Read the model definition and answer for the solid it produces. Units are mm, in the model's axes. Face numbers are marked on the shaded views. A direction names the side the tool comes from. Give positions to 0.01 mm unless a question says otherwise; leave off trailing zeros. Write each loop counter-clockwise with the first axis right and the second up, starting at its lowest first coordinate (ties: lowest second). Pieces come first, ordered by that corner, then holes. Notation, with made-up numbers: (45.5, 50.5) -> (101.5, 50.5) arc R26 cw to (101.5, 81.5) -> close; hole circle Ø6 at (-8, 85). An arc over 180 degrees is marked (long way). Answer as CSV lines item,"result". Start each with the question number.
1. For a pull along Y with two mould halves and no side action, classify the marked faces 3, 4 and 5 as pulls with the +Y half, pulls with the -Y half, needs draft (parallel to the pull), parting line crosses it, or undercut.
2. The part is cut by section A-A, the plane x = 0. Determine the outline of the cut face in (y, z).
3. The part is cut by section B-B, the plane y = 8.5. Determine the outline of the cut face in (x, z), and give its area (3 significant figures).
4. A tool of negligible diameter and unlimited length cuts with its end or side. For the marked faces 1 and 2, from which of +Z, -Z, +X, -X, +Y, -Y can it reach the whole face along a straight path? Write none if from no direction.
5. Given pin 1 (5.5 mm diameter, centred on x = -15.5, y = -15.5, fed in from +Z); pin 2 (1.5 mm diameter, centred on x = -18, z = 5, fed in from -Y); pin 3 (4.5 mm diameter, centred on x = 15.5, y = 15.5, fed in from -Z); pin 4 (1.7 mm diameter, centred on y = 3, z = 6, fed in from +X), each flat-ended and moving along its own axis, determine where each tip first touches the part or whether it passes through.
6. The part is cut by section D-D, the plane y = -16. Determine the outline of the cut face in (x, z).
7. Find the intervals of material crossed by line 1 (Y direction, x = -15.5, z = 1.15); line 2 (Y direction, x = 0, z = 0.85); line 3 (X direction, y = 6.5, z = 3.75), in increasing order.
8. The part is cut by section C-C, the plane x = -15.5. Determine the outline of the cut face in (y, z), and give its area (4 significant figures).
from build123d import *

# Parameters (mm, degrees)
SKETCH_W        = 42.3
SKETCH_H        = 40.3
SKETCH_R        = 12
SKETCH_R_2      = 1.7
PAD_DEPTH       = 3
CHAMFER_SIZE    = 5
SKETCH001_W     = 5
SKETCH001_H     = 20
PAD001_DEPTH    = 5
SKETCH002_R     = 1.7
POCKET_DEPTH    = 42.301
POCKET001_DEPTH = 1.5


with BuildPart() as part:
    # Sketch → Pad (new body)
    with BuildSketch(Plane.XY):
        Rectangle(SKETCH_W, SKETCH_H)
        Circle(SKETCH_R, mode=Mode.SUBTRACT)
        with Locations((-15.5, 15.5)):
            Circle(SKETCH_R_2, mode=Mode.SUBTRACT)
        with Locations((-15.5, -15.5)):
            Circle(SKETCH_R_2, mode=Mode.SUBTRACT)
        with Locations((15.5, -15.5)):
            Circle(SKETCH_R_2, mode=Mode.SUBTRACT)
        with Locations((15.5, 15.5)):
            Circle(SKETCH_R_2, mode=Mode.SUBTRACT)
    extrude(amount=PAD_DEPTH)

    # Chamfer
    chamfer_edges = [part.edges().sort_by_distance(p)[0] for p in [
        (21.15, -20.15, 1.5),
        (-21.15, -20.15, 1.5),
        (21.15, 20.15, 1.5),
        (-21.15, 20.15, 1.5),
    ]]
    chamfer(chamfer_edges, length=CHAMFER_SIZE)

    # Sketch001 (on Face5 of Chamfer) → Pad001 (join)
    with BuildSketch(Plane.XY.offset(3)):
        with Locations((-18.65, 0)):
            Rectangle(SKETCH001_W, SKETCH001_H)
    extrude(amount=PAD001_DEPTH)

    # Sketch002 (on Face19 of Pad001) → Pocket (cut, through all)
    with BuildSketch(Plane(origin=(-21.15, 0, 0), x_dir=(0, -1, 0), z_dir=(-1, 0, 0))):
        with Locations((-4.5, 5)):
            Circle(SKETCH002_R)
        with Locations((4.5, 5)):
            Circle(SKETCH002_R)
    extrude(amount=-POCKET_DEPTH, mode=Mode.SUBTRACT)

    # Sketch003 (on DatumPlane) → Pocket001 (cut, symmetric)
    with BuildSketch(Plane(origin=(-18.65, 0, 0), x_dir=(0, -1, 0), z_dir=(-1, 0, 0))):
        Polygon((4.5, 1.65), (7.401185, 3.325), (7.401185, 13.325), (1.598815, 13.325), (1.598815, 3.325), align=None)
        Polygon((-4.5, 1.65), (-1.598815, 3.325), (-1.598815, 13.325), (-7.401185, 13.325), (-7.401185, 3.325), align=None)
    extrude(amount=POCKET001_DEPTH, both=True, mode=Mode.SUBTRACT)


solid = part.part
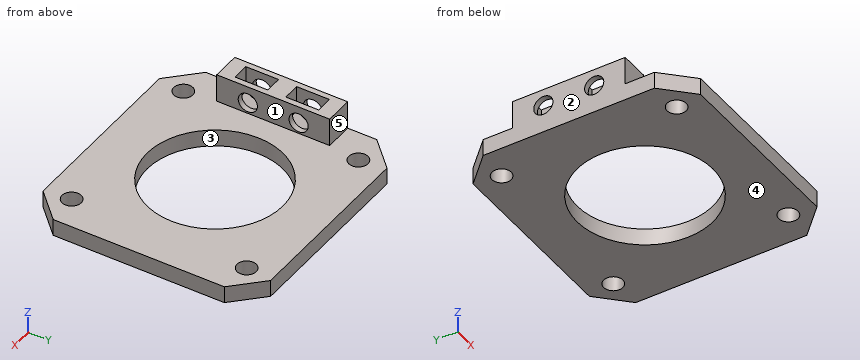
Results found:
1,face 3,"undercut"
1,face 4,"needs draft"
1,face 5,"pulls with the +Y half"
2,outline,"(-20.15, 0) -> (-12, 0) -> (-12, 3) -> (-20.15, 3) -> close; (12, 0) -> (20.15, 0) -> (20.15, 3) -> (12, 3) -> close"
3,outline,"(-21.15, 0) -> (-8.47, 0) -> (-8.47, 3) -> (-16.15, 3) -> (-16.15, 8) -> (-21.15, 8) -> close; (8.47, 0) -> (21.15, 0) -> (21.15, 3) -> (8.47, 3) -> close"
3,area,"101 mm²"
4,face 1,"+Z, +X, +Y, -Y"
4,face 2,"+Z, -Z, -X, +Y, -Y"
5,pin 1,"stops at z = 3"
5,pin 2,"stops at y = -10"
5,pin 3,"stops at z = 0"
5,pin 4,"stops at x = -16.15"
6,outline,"(-20.3, 0) -> (-17.12, 0) -> (-17.12, 3) -> (-20.3, 3) -> close; (-13.88, 0) -> (13.88, 0) -> (13.88, 3) -> (-13.88, 3) -> close; (17.12, 0) -> (20.3, 0) -> (20.3, 3) -> (17.12, 3) -> close"
7,line 1,"y = -20.15 to -17.2, -13.8 to 13.8, 17.2 to 20.15"
7,line 2,"y = -20.15 to -12, 12 to 20.15"
7,line 3,"x = -21.15 to -20.15, -17.15 to -16.15"
8,outline,"(-20.15, 0) -> (-17.2, 0) -> (-17.2, 3) -> (-20.15, 3) -> close; (-13.8, 0) -> (13.8, 0) -> (13.8, 3) -> (-13.8, 3) -> close; (17.2, 0) -> (20.15, 0) -> (20.15, 3) -> (17.2, 3) -> close"
8,area,"100.5 mm²"
